from build123d import *

# Parameters (mm, degrees)
SKETCH1_W           = 19.05
SKETCH1_H           = 76.2
SKETCH1_R           = 1.5875
SKETCH1_R_2         = 3.4925
SKETCH1_W_2         = 12.827
SKETCH1_H_2         = 3.302
BOSS_EXTRUDE1_DEPTH = 3.175
FILLET1_R           = 8.89
FILLET2_R           = 8.89


with BuildPart() as part:
    # Sketch1 → Boss-Extrude1 (new body)
    with BuildSketch(Plane(origin=(0, 0, 0), x_dir=(1, 0, 0), z_dir=(0, 1, 0))):
        Rectangle(SKETCH1_W, SKETCH1_H)
        with Locations((0, 25.4)):
            Circle(SKETCH1_R, mode=Mode.SUBTRACT)
        with Locations((0, -31.75)):
            Circle(SKETCH1_R_2, mode=Mode.SUBTRACT)
        with Locations((0, -8.001)):
            Rectangle(SKETCH1_W_2, SKETCH1_H_2, mode=Mode.SUBTRACT)
    extrude(amount=BOSS_EXTRUDE1_DEPTH)

    # Fillet1
    fillet1_edges = [part.edges().sort_by_distance(p)[0] for p in [
        (9.525, 1.5875, -38.1),
    ]]
    fillet(fillet1_edges, radius=FILLET1_R)

    # Fillet2
    fillet2_edges = [part.edges().sort_by_distance(p)[0] for p in [
        (-9.525, 1.5875, -38.1),
    ]]
    fillet(fillet2_edges, radius=FILLET2_R)


solid = part.part
Geometry: final body of the model. Coordinates: model frame, mm. A direction names the side the tool comes from. Give positions to 0.01 mm unless a question says otherwise; leave off trailing zeros. Loops run counter-clockwise (first coordinate to the right, second up) from the corner with the lowest first, then second, coordinate; pieces in that order, holes last. Notation, with made-up numbers: (29, -20) - (44, -20) arc R28 cw to (44, 13) - close; hole circle Ø1 at (-33.5, 51.5). An arc over 180 degrees is marked (long way). Answer as CSV lines item,"result". Start each with the question number.
1. Pin query (flat end, axial travel): P1, Ø1.6, axis at x = 3, y = 2, coming from the -Z side. Return the tip coordinate at first contact, or that it passes through.
2. Reachability of faces 1 (the face through (0, 2, -38.1)), 2 (the face through (0, 2, 9.652)) from +Z, -Z, +X, -X, +Y, -Y: full face, straight path, thin tool, end or side. Return the list, or none.
3. Section D-D, the plane x = -5. Return loops of the section in (y, z) (3 decimals).
4. Section A-A, the plane z = 31.75. Return loops of the section in (x, y) (1 decimal), plus the area to 3 significant figures.
5. Ray query, L1, parallel to Z at x = 0, y = 1.9; L2, parallel to X at y = 2.25, z = 9.5 (1 decimal); L3, parallel to X at y = 2.05, z = 31.75 (1 decimal). Return the intervals inside material, ascending.
6. Draft query along X for faces 3 (the face through (-6.414, 2, 8)), 4 (the face through (9.525, 2, 5)), 5 (the face through (0, 2, 38.1)). Return one class per face: released by +X, released by -X, zero draft, split by the parting line, or undercut.
7. Section B-B, the plane x = 0. Give the number of separate pieces and of enclosed holes in the cut face, plus the area to 3 significant figures.
Answers:
1,P1,"stops at z = -37.96"
2,face 1,"-Z, +X, -X, +Y, -Y"
2,face 2,"+Y, -Y"
3,outline,"(0, -36.955) - (3.175, -36.955) - (3.175, 6.35) - (0, 6.35) - close; (0, 9.652) - (3.175, 9.652) - (3.175, 38.1) - (0, 38.1) - close"
4,outline,"(-9.5, 0) - (-3.5, 0) - (-3.5, 3.2) - (-9.5, 3.2) - close; (3.5, 0) - (9.5, 0) - (9.5, 3.2) - (3.5, 3.2) - close"
4,area,"38.3 mm2"
5,L1,"z = -38.1 to -26.99, -23.81 to 6.35, 9.65 to 28.26, 35.24 to 38.1"
5,L2,"x = -9.5 to -6.4, 6.4 to 9.5"
5,L3,"x = -9.5 to -3.5, 3.5 to 9.5"
6,face 3,"undercut"
6,face 4,"released by +X"
6,face 5,"zero draft"
7,separate pieces,"4"
7,enclosed holes,"0"
7,area,"199 mm2"
